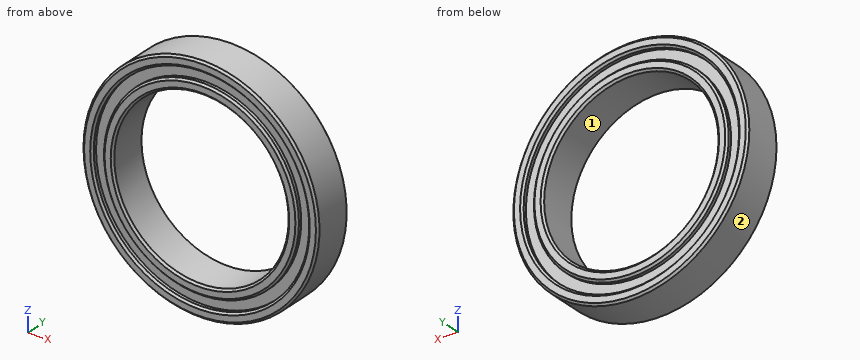
Autodesk Inventor part; units mm, degrees
ref_plane "YZ Plane" through (0, 0, 0) normal (1, 0, 0) x (0, 1, 0)
ref_plane "XZ Plane" through (0, 0, 0) normal (0, 1, 0) x (-1, 0, 0)
ref_plane "XY Plane" through (0, 0, 0) normal (0, 0, 1) x (1, 0, 0)
sketch "Эскиз1" plane through (0, 0, 0) normal (0, 1, 0) x (-1, 0, 0)
  circle A0 centre (0, 0) radius 11.5
  circle A1 centre (0, 0) radius 8.5
  dimension "d0" = 23
  dimension "d1" = 17
extrude "Выдавливание1" add sketch "Эскиз1" along normal blind 4
sketch "Эскиз2" plane through (0, 4, 0) normal (0, 1, 0) x (1, 0, 0)
  circle A0 centre (0, 0) radius 9.5
  circle A1 centre (0, 0) radius 10.5
  circle A2 centre (0, 0) radius 11.5
  circle A3 centre (0, 0) radius 8.5
  dimension "d4" = 1
  dimension "d5" = 1
extrude "Выдавливание2" cut sketch "Эскиз2" against normal blind 0.5 contours A1
sketch "Эскиз3" plane through (0, 0, 0) normal (0, -1, 0) x (1, 0, 0)
  circle A0 centre (0, 0) radius 9.5
  circle A1 centre (0, 0) radius 10.5
extrude "Выдавливание3" cut sketch "Эскиз3" against normal blind 0.5
chamfer "Фаска1" distance 0.2 angle 45 8 edges at (-9.5, 0, 0) (8.5, 0, 0) (-10.5, 0, 0) (11.5, 0, 0) (11.5, 4, 0) (-10.5, 4, 0) (-9.5, 4, 0) (8.5, 4, 0)
properties part number "Подшипник 17x23x4" material "Титан"
Geometry check sheet. Reference: the model listing, model coordinates, mm. Face numbers are marked on the shaded views. Give positions to 0.01 mm unless a question says otherwise; leave off trailing zeros. Loops run counter-clockwise (first coordinate to the right, second up) from the corner with the lowest first, then second, coordinate; pieces in that order, holes last. Notation, with made-up numbers: M -27.5,-23 L -7.5,-23 A20 ccw -7.5,9 Z; hole C 24.5,-26 d4. An arc over 180 degrees is marked long. Write item = value, one per line.
(1) Material ranges on line 1 (Z direction, x = 0, y = 3.7); line 2 (X direction, y = 1.55, z = -0.25); line 3 (Z direction, x = 2.75, y = 0.3), recorded low to high. Write a range as [from, to].
Answer below:
line_1 = [-11.5, -10.5], [-9.5, -8.5], [8.5, 9.5], [10.5, 11.5]
line_2 = [-11.5, -8.5], [8.5, 11.5]
line_3 = [-11.17, -10.13], [-9.09, -8.04], [8.04, 9.09], [10.13, 11.17]
(2) Sectioned sample at A-A, the plane y = 1.25. Record the cut outline in (x, z), plus the area to 3 significant figures.
Answer below:
outline = C 0,0 d23; hole C 0,0 d17
area = 188 mm2
(3) Gauge pin test, flat ends, axial feed: pin 1 Ø2 at (x, y) = (4, 3) entering from -Z; pin 2 Ø12 at (x, z) = (-0.5, 0.5) entering from -Y; pin 3 Ø1 at (y, z) = (2, 6.5) entering from +X. Record the tip position at first contact, or that the pin passes through.
Answer below:
pin_1 = -11.1
pin_2 = through
pin_3 = 9.81
(4) Release check for a two-part mould opening along Z. For the marked faces 1 and 2 record: released by +Z, released by -Z, zero draft, split by the parting line, or undercut.
Answer below:
face_1 = undercut
face_2 = split by the parting line
